```python
from build123d import *

# Parameters (mm, degrees)
SKETCH1_W                                = 60
SKETCH1_H                                = 12
BOSS_EXTRUDE1_DEPTH                      = 11.5
SKETCH4_W                                = 60
SKETCH4_H                                = 8
BOSS_EXTRUDE2_DEPTH                      = 17.5
SKETCH9_W                                = 12
SKETCH9_H                                = 11.5
BOSS_EXTRUDE3_DEPTH                      = 60
CBORE_FOR_M5_PAN_HEAD_SCREW2_D           = 5.8
CBORE_FOR_M5_PAN_HEAD_SCREW2_DEPTH       = 8.2
CBORE_FOR_M5_PAN_HEAD_SCREW2_CBORE_D     = 11
CBORE_FOR_M5_PAN_HEAD_SCREW2_CBORE_DEPTH = 3.7
CBORE_FOR_M5_PAN_HEAD_SCREW2_TIP         = 1.742495795
F_5_0MM_DOWEL_HOLE7_D                    = 5
F_5_0MM_DOWEL_HOLE7_DEPTH                = 9
F_5_0MM_DOWEL_HOLE7_TIP                  = 1.502151548
F_5_0MM_DOWEL_HOLE8_D                    = 5
F_5_0MM_DOWEL_HOLE8_DEPTH                = 9
F_5_0MM_DOWEL_HOLE8_TIP                  = 1.502151548
M5_TAPPED_HOLE2_D                        = 4.2
M5_TAPPED_HOLE2_DEPTH                    = 12.4
M5_TAPPED_HOLE2_TIP                      = 1.2618073
M5_TAPPED_HOLE3_D                        = 4.2
M5_TAPPED_HOLE3_DEPTH                    = 12.4
M5_TAPPED_HOLE3_TIP                      = 1.2618073


with BuildPart() as part:
    # Sketch1 → Boss-Extrude1 (new body)
    with BuildSketch(Plane(origin=(0, 0, 0), x_dir=(1, 0, 0), z_dir=(0, 1, 0))):
        with Locations((30, 6)):
            Rectangle(SKETCH1_W, SKETCH1_H)
    extrude(amount=BOSS_EXTRUDE1_DEPTH)

    # Sketch4 → Boss-Extrude2 (add)
    with BuildSketch(Plane(origin=(0, 0, 0), x_dir=(1, 0, 0), z_dir=(0, 1, 0))):
        with Locations((30, 4)):
            Rectangle(SKETCH4_W, SKETCH4_H)
    extrude(amount=BOSS_EXTRUDE2_DEPTH)

    # Sketch9 → Boss-Extrude3 (add)
    with BuildSketch(Plane(origin=(0, 0, 0), x_dir=(0, 0, -1), z_dir=(1, 0, 0))):
        with Locations((6, 23.25)):
            Rectangle(SKETCH9_W, SKETCH9_H)
    extrude(amount=BOSS_EXTRUDE3_DEPTH)

    # CBORE for M5 Pan Head Screw2
    with Locations(Plane.XY):
        with Locations((50, 14.5), (10, 14.5)):
            CounterBoreHole(CBORE_FOR_M5_PAN_HEAD_SCREW2_D / 2, CBORE_FOR_M5_PAN_HEAD_SCREW2_CBORE_D / 2, CBORE_FOR_M5_PAN_HEAD_SCREW2_CBORE_DEPTH, depth=CBORE_FOR_M5_PAN_HEAD_SCREW2_DEPTH)
            with Locations((0, 0, -(CBORE_FOR_M5_PAN_HEAD_SCREW2_DEPTH + CBORE_FOR_M5_PAN_HEAD_SCREW2_TIP / 2))):  # 118° drill point
                Cone(0, CBORE_FOR_M5_PAN_HEAD_SCREW2_D / 2, CBORE_FOR_M5_PAN_HEAD_SCREW2_TIP, mode=Mode.SUBTRACT)

    # Ø5.0mm Dowel Hole7
    with Locations(Plane(origin=(0, 29, 0), x_dir=(1, 0, 0), z_dir=(0, 1, 0))):
        with Locations((7.5, 6)):
            Hole(F_5_0MM_DOWEL_HOLE7_D / 2, depth=F_5_0MM_DOWEL_HOLE7_DEPTH)
            with Locations((0, 0, -(F_5_0MM_DOWEL_HOLE7_DEPTH + F_5_0MM_DOWEL_HOLE7_TIP / 2))):  # 118° drill point
                Cone(0, F_5_0MM_DOWEL_HOLE7_D / 2, F_5_0MM_DOWEL_HOLE7_TIP, mode=Mode.SUBTRACT)

    # Ø5.0mm Dowel Hole8
    with Locations(Plane(origin=(0, 29, 0), x_dir=(1, 0, 0), z_dir=(0, 1, 0))):
        with Locations((52.5, 6)):
            Hole(F_5_0MM_DOWEL_HOLE8_D / 2, depth=F_5_0MM_DOWEL_HOLE8_DEPTH)
            with Locations((0, 0, -(F_5_0MM_DOWEL_HOLE8_DEPTH + F_5_0MM_DOWEL_HOLE8_TIP / 2))):  # 118° drill point
                Cone(0, F_5_0MM_DOWEL_HOLE8_D / 2, F_5_0MM_DOWEL_HOLE8_TIP, mode=Mode.SUBTRACT)

    # M5 Tapped Hole2
    with Locations(Plane(origin=(0, 29, 0), x_dir=(1, 0, 0), z_dir=(0, 1, 0))):
        with Locations((16, 5.948108633)):
            Hole(M5_TAPPED_HOLE2_D / 2, depth=M5_TAPPED_HOLE2_DEPTH)
            with Locations((0, 0, -(M5_TAPPED_HOLE2_DEPTH + M5_TAPPED_HOLE2_TIP / 2))):  # 118° drill point
                Cone(0, M5_TAPPED_HOLE2_D / 2, M5_TAPPED_HOLE2_TIP, mode=Mode.SUBTRACT)

    # M5 Tapped Hole3
    with Locations(Plane(origin=(0, 29, 0), x_dir=(1, 0, 0), z_dir=(0, 1, 0))):
        with Locations((44, 5.948108633)):
            Hole(M5_TAPPED_HOLE3_D / 2, depth=M5_TAPPED_HOLE3_DEPTH)
            with Locations((0, 0, -(M5_TAPPED_HOLE3_DEPTH + M5_TAPPED_HOLE3_TIP / 2))):  # 118° drill point
                Cone(0, M5_TAPPED_HOLE3_D / 2, M5_TAPPED_HOLE3_TIP, mode=Mode.SUBTRACT)


solid = part.part
```
Read the model definition and answer for the solid it produces. Units are mm, in the model's axes. A direction names the side the tool comes from. Give positions to 0.01 mm unless a question says otherwise; leave off trailing zeros. Order: outer loops, then holes, each group sorted by start corner. A loop starts at its lowest first (then second) coordinate and runs counter-clockwise, first axis right, second up. Notation, with made-up numbers: (-31, 4.5) -> (28, 4.5) arc R31 cw to (28, 33.5) -> close; hole circle Ø1 at (81.25, -29). An arc over 180 degrees is marked (long way). One line per item, written item: value. Start each with the question number.
(1) A tool of negligible diameter and unlimited length cuts with its end or side. For faces 5 (the flat face through (12, 12, -3.7)), 6 (the flat face through (30, 29, -6)), 7 (the flat face through (30, 14, -8)), 8 (the cylindrical face through (9, 24, -8)), from which of +Z, -Z, +X, -X, +Y, -Y can it reach the whole face along a straight path? Write none if from no direction.
(2) The part is cut by section C-C (y = 22). Determine the outline of the cut face in (x, z).
(3) Flat-ended cylindrical pins translate along their axes: P1, Ø3.5, axis at x = 52, y = 15.5, coming from the +Z side; P2, Ø4, axis at x = 30, z = -6.5, coming from the -Y side; P3, Ø3, axis at x = 52.5, z = -6, coming from the +Y side; P4, Ø5, axis at x = 50, y = 14.5, coming from the +Z side. Find the tip coordinate at first contact, or state that the pin passes through.
(4) Straight lines are drawn through the part: L1, parallel to Y at x = 4, z = -9.5; L2, parallel to X at y = 12.5, z = -6; L3, parallel to Z at x = 52.5, y = 22.5. For each, find the intervals that lie inside material, in ascending order.
(5) The part is cut by section D-D (z = -4.5). State how many separate pieces and enclosed holes the cut face has, and give its area (3 significant figures).
(6) The part is cut by section B-B (z = -1.5). Determine the outline of the cut face in (x, y).
(7) For a pull along X with two mould halves and no side action, classify faces 1 (the conical face through (52.9, 18.76, -5.83)), 2 (the flat face through (52, 12, -3.7)), 3 (the flat face through (60, 15, -6)), 4 (the flat face through (30, 6, -12)) as released by +X, released by -X, zero draft, split by the parting line, or undercut.
(8) The part is cut by section A-A (y = 14.5). Determine the outline of the cut face in (x, z).
Taken from the geometry:
1. face 5: +Z
1. face 6: +Z, -Z, +X, -X, +Y
1. face 7: -Z, +X, -X
1. face 8: +Y
2. outline: (0, -12) -> (60, -12) -> (60, 0) -> (0, 0) -> close; hole circle Ø5 at (7.5, -6); hole circle Ø4.2 at (16, -5.95); hole circle Ø4.2 at (44, -5.95); hole circle Ø5 at (52.5, -6)
3. P1: z = -3.7
3. P2: y = 0
3. P3: y = 19.4
3. P4: through
4. L1: 0 to 11.5, 17.5 to 29
4. L2: 0 to 7.9, 12.1 to 47.9, 52.1 to 60
4. L3: -12 to -8.5, -3.5 to 0
5. separate pieces: 1
5. enclosed holes: 2
5. area: 1,540 mm^2
6. outline: (0, 0) -> (60, 0) -> (60, 29) -> (0, 29) -> close; hole circle Ø11 at (10, 14.5); hole circle Ø11 at (50, 14.5)
7. face 1: undercut
7. face 2: undercut
7. face 3: released by +X
7. face 4: zero draft
8. outline: (0, -8) -> (7.1, -8) -> (7.1, -3.7) -> (4.5, -3.7) -> (4.5, 0) -> (0, 0) -> close; (12.9, -8) -> (47.1, -8) -> (47.1, -3.7) -> (44.5, -3.7) -> (44.5, 0) -> (15.5, 0) -> (15.5, -3.7) -> (12.9, -3.7) -> close; (52.9, -8) -> (60, -8) -> (60, 0) -> (55.5, 0) -> (55.5, -3.7) -> (52.9, -3.7) -> close
